Answer from the drawing. Dimensions are ordinates in mm from the lowest x, y and z of the part. Round coordinates to 2 decimals unless told otherwise and drop trailing zeros. Loops run counter-clockwise (first coordinate to the right, second up) from the corner with the lowest first, then second, coordinate; pieces in that order, holes last. Notation, with made-up numbers: (55, -39) - (108, -39) arc R10 ccw to (108, -33) - close; hole circle Ø5 at (80, 58.25). An arc over 180 degrees is marked (long way). Answer as CSV lines item,"result". Start each with the question number.
Q1. Straight lines are drawn through the part: L1, parallel to Y at x = 82.55, z = 1.95 (3 decimals); L2, parallel to X at y = 4.5, z = 2.2; L3, parallel to Y at x = 44.45, z = 1.8 (3 decimals). For each, find the intervals that lie inside material, in ascending order. Write a range as [from, to].
Q2. Section D-D on z = 1.35 is taken. Write down the section's boundary in (x, y) (3 decimals), then the cut area to 3 significant figures.
Q3. This flat-tipped pin is pushed along its axis until it touches: pin 1 Ø8.5 at (x, y) = (82.55, 6.35) entering from -Z. Where does it stop, or does it pass through?
Q4. Section C-C on x = 44.45 is taken. Write down the section's boundary in (y, z) (3 decimals), then the cut area to 3 significant figures.
Q5. Section A-A on x = 6.35 is taken. Write down the section's boundary in (y, z) (3 decimals).
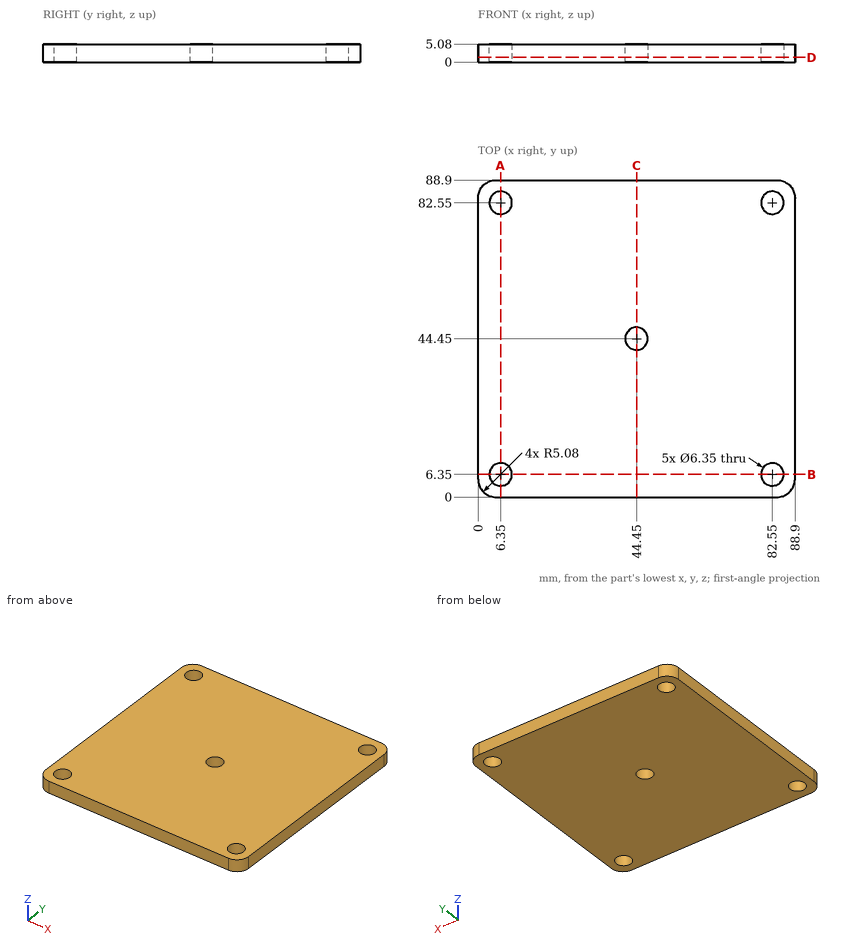
Findings:
1,L1,"y = [0, 3.175], [9.525, 79.375], [85.725, 88.9]"
1,L2,"x = [0.03, 3.77], [8.93, 79.97], [85.13, 88.87]"
1,L3,"y = [0, 41.275], [47.625, 88.9]"
2,outline,"(0, 5.08) arc R5.08 ccw to (5.08, 0) - (83.82, 0) arc R5.08 ccw to (88.9, 5.08) - (88.9, 83.82) arc R5.08 ccw to (83.82, 88.9) - (5.08, 88.9) arc R5.08 ccw to (0, 83.82) - close; hole circle Ø6.35 at (6.35, 6.35); hole circle Ø6.35 at (6.35, 82.55); hole circle Ø6.35 at (44.45, 44.45); hole circle Ø6.35 at (82.55, 6.35); hole circle Ø6.35 at (82.55, 82.55)"
2,area,"7,720 mm^2"
3,pin 1,"stops at z = 0"
4,outline,"(0, 0) - (41.275, 0) - (41.275, 5.08) - (0, 5.08) - close; (47.625, 0) - (88.9, 0) - (88.9, 5.08) - (47.625, 5.08) - close"
4,area,"419 mm^2"
5,outline,"(0, 0) - (3.175, 0) - (3.175, 5.08) - (0, 5.08) - close; (9.525, 0) - (79.375, 0) - (79.375, 5.08) - (9.525, 5.08) - close; (85.725, 0) - (88.9, 0) - (88.9, 5.08) - (85.725, 5.08) - close"
